from build123d import *

# Parameters (mm, degrees)
ESBO_O1_W                = 36
ESBO_O1_H                = 36
RESSALTO_EXTRUS_O1_DEPTH = 1
RESSALTO_EXTRUS_O1_TAPER = 60
RESSALTO_EXTRUS_O2_DEPTH = 3
ESBO_O2_W                = 32
ESBO_O2_H                = 7
RESSALTO_EXTRUS_O3_DEPTH = 1
RESSALTO_EXTRUS_O3_TAPER = 60


with BuildPart() as part:
    # Esbo_o1 → Ressalto-extrus_o1 (new body)
    with BuildSketch(Plane.XY):
        with Locations((0, 15)):
            Rectangle(ESBO_O1_W, ESBO_O1_H)
    extrude(amount=RESSALTO_EXTRUS_O1_DEPTH, taper=RESSALTO_EXTRUS_O1_TAPER)

    # Esbo_o1_4 → Ressalto-extrus_o2 (add)
    with BuildSketch(Plane.XY):
        Polygon((16, 31), (16, -1), (16, -3), (18, -3), (18, 33), (0, 33), (-18, 33), (-18, -3), (-16, -3), (-16, -1), (-16, 31), (0, 31), align=None)
    extrude(amount=-RESSALTO_EXTRUS_O2_DEPTH)

    # Esbo_o2 → Ressalto-extrus_o3 (add)
    with BuildSketch(Plane(origin=(0, 0, -3), x_dir=(-1, 0, 0), z_dir=(0, 0, -1))):
        Polygon((18, -3), (18, 33), (-18, 33), (-18, -3), (-16, -3), (16, -3), align=None)
        with Locations((0, 7.5)):
            Rectangle(ESBO_O2_W, ESBO_O2_H, mode=Mode.SUBTRACT)
    extrude(amount=RESSALTO_EXTRUS_O3_DEPTH, taper=RESSALTO_EXTRUS_O3_TAPER)


solid = part.part
The listing builds one solid part. Answer for the finished solid, in the listing's coordinates (mm). A direction names the side the tool comes from. Round coordinates to 2 decimals unless told otherwise and drop trailing zeros. Order: outer loops, then holes, each group sorted by start corner. A loop starts at its lowest first (then second) coordinate and runs counter-clockwise, first axis right, second up. Notation, with made-up numbers: (-28, 22) - (25, 22) arc R38 ccw to (25, 61) - close; hole circle Ø2 at (27.25, 6). An arc over 180 degrees is marked (long way). Write item = value, one per line. Start each with the question number.
1) For faces 5 (the flat face through (0, 33, -1)), 6 (the flat face through (0, 31, -1)), determine the directions among +Z, -Z, +X, -X, +Y, -Y from which every point of the face is accessible in a straight line to the end or side of a thin tool.
2) For a pull along X with two mould halves and no side action, classify faces 1 (the flat face through (16, 14, -1)), 2 (the flat face through (17.15, 15.25, 0.49)), 3 (the flat face through (0.25, -2.15, 0.49)), 4 (the flat face through (0, 21, -3)) as released by +X, released by -X, zero draft, split by the parting line, or undercut.
3) Given pin 1 (0.9 mm diameter, centred on x = -3, z = -1, fed in from -Y), flat-ended and moving along its own axis, determine where the tip first touches the part or whether it passes through.
4) Straight lines are drawn through the part: L1, parallel to X at y = 5, z = -0.5; L2, parallel to Z at x = -12.5, y = 13.5; L3, parallel to Y at x = -1.5, z = -1.4. For each, find the intervals that lie inside material, in ascending order.
5) Section A-A, the plane z = -1.8 is taken. Write down the section's boundary in (x, y).
Results list:
q1.face_5 = +Z, -Z, +X, -X, +Y
q1.face_6 = -Y
q2.face_1 = undercut
q2.face_2 = released by +X
q2.face_3 = zero draft
q2.face_4 = undercut
q3.pin_1 = 31
q4.L1 = -18 to -16, 16 to 18
q4.L2 = -4 to -3, 0 to 1
q4.L3 = 31 to 33
q5.outline = (-18, -3) - (-16, -3) - (-16, 31) - (16, 31) - (16, -3) - (18, -3) - (18, 33) - (-18, 33) - close
